For this review, take the finished solid that the model builds, in its own axes (mm). Face numbers are marked on the shaded views. Coordinates: 2 decimals unless noted, no trailing zeros. Loops run counter-clockwise (first coordinate to the right, second up) from the corner with the lowest first, then second, coordinate; pieces in that order, holes last. Notation, with made-up numbers: (-2, 40.25) - (51, 40.25) arc R23 ccw to (51, 49.25) - close; hole circle Ø3 at (30.5, 49.25). An arc over 180 degrees is marked (long way). Answer as a JSON object with one key per item and string values. Group by question number.
Item 1: We need section A-A (x = 0.4). Give the boundary of the cut face in (y, z).
Item 2: Clearance check with flat-ended pins moving along their axes: pin 1 (1.9 mm diameter, centred on y = 8, z = 90, fed in from -X); pin 2 (2 mm diameter, centred on x = 2.5, y = 0.5, fed in from -Z). State where each tip first meets the part, or that it passes through.
Item 3: We need section C-C (z = 108). Give the boundary of the cut face in (x, y), then the cut area to 3 significant figures.
Item 4: To check wall thickness, follow line 1 (Z direction, x = 3.1, y = 9); line 2 (Z direction, x = 2.05, y = 8); line 3 (Y direction, x = 1.2, z = 108). State the ranges of each line that lie inside material, in increasing order.
Item 5: Mouldability with a two-part tool opening along Y and no side actions: class the marked faces 1, 2 and 3 as released by +Y, released by -Y, zero draft, split by the parting line, or undercut.
Item 6: We need section B-B (y = 8). Give the boundary of the cut face in (x, z).
Item 7: We need section D-D (y = 2.5). Give the boundary of the cut face in (x, z).
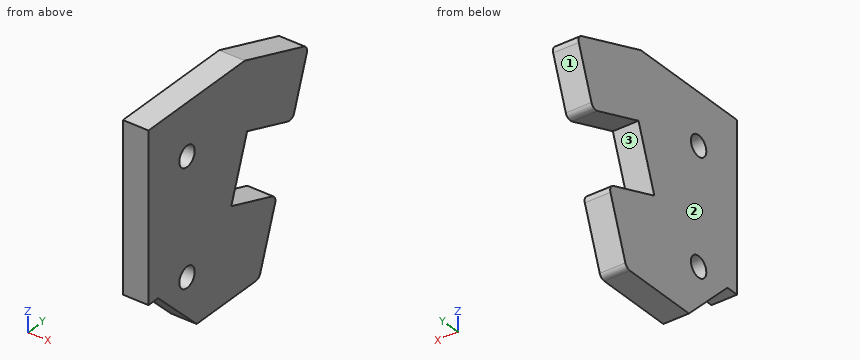
Autodesk Fusion 360 part; units mm, degrees
sketch "スケッチ1" plane through (0, 0, 0) normal (1, 0, 0) x (0, 0, -1)
  line L0 (-116, 0) -> (-116, 20)
  line L1 (-116, 20) -> (-111.3943, 33.2207)
  line L2 (-111.3943, 33.2207) -> (-101.951, 29.931)
  line L3 (-101.951, 29.931) -> (-105.2407, 20.4876)
  line L4 (-105.2407, 20.4876) -> (-95.7973, 17.1978)
  line L5 (-14, 252) -> (0, 252)
  line L6 (-95.7973, 17.1978) -> (-79.3485, 64.4147)
  line L7 (-79.3485, 64.4147) -> (-65.1834, 59.4801)
  line L8 (-65.1834, 59.4801) -> (-63.8675, 63.2574)
  line L9 (-63.8675, 63.2574) -> (-78.0326, 68.1921)
  line L10 (-78.0326, 68.1921) -> (-38.5555, 181.5127)
  line L11 (-38.5555, 181.5127) -> (-24.3904, 176.578)
  line L12 (-24.3904, 176.578) -> (-23.0745, 180.3554)
  line L13 (-23.0745, 180.3554) -> (-37.2396, 185.29)
  line L14 (-37.2396, 185.29) -> (-14, 252)
  line L15 (-116, 0) -> (-70, 0)
  line L16 (-70, 0) -> (-70, -4)
  line L17 (-70, -4) -> (-50, -4)
  line L18 (-50, -4) -> (-50, 0)
  line L19 (-50, 0) -> (0, 0)
  line L20 (0, 252) -> (0, 165)
  line L21 (0, 165) -> (4, 165)
  line L22 (4, 165) -> (4, 145)
  line L23 (4, 145) -> (0, 145)
  line L24 (0, 145) -> (0, 0)
  line L25 (4, 155) -> (-13.5, 155)
  line L26 (-60, -4) -> (-60, 13.5)
  line L27 (-64.1481, 77.6509) -> (-33.5533, 165.4743)
  line L28 (-10, 10) -> (-30, 10)
  line L29 (-30, 10) -> (-30, 30)
  line L30 (-30, 30) -> (-10, 30)
  line L31 (-10, 30) -> (-10, 10)
  line L32 (-108, 8) -> (-90, 8)
  line L33 (-102.8799, 19.6651) -> (-98.1582, 18.0203)
  line L34 (-98.1582, 18.0203) -> (-99.1451, 15.1873)
  line L35 (-99.1451, 15.1873) -> (-103.8668, 16.8321)
  line L36 (-103.8668, 16.8321) -> (-102.8799, 19.6651)
  line L37 (-92.5076, 26.6412) -> (-82, 22.9807)
  line L38 (-82, 22.9807) -> (-82, 0)
  line L39 (-90, 0) -> (-90, 2)
  line L40 (-90, 2) -> (-82, 10)
  dimension "d1" = 116
  dimension "d2" = 20
  dimension "d3" = 14
  dimension "d4" = 10
  dimension "d5" = 10
  dimension "d6" = 10
  dimension "d9" = 14
  dimension "d11" = 252
  dimension "d12" = 248.642
  dimension "d13" = 4
  dimension "d14" = 4
  dimension "d15" = 120
  dimension "d16" = 50
  dimension "d17" = 15
  dimension "d18" = 20
  dimension "d19" = 4
  dimension "d20" = 50
  dimension "d21" = 4
  dimension "d22" = 20
  dimension "d23" = 145
  dimension "d24" = 17.5
  dimension "d25" = 17.5
  dimension "d31" = 10
  dimension "d32" = 13.5
  dimension "d33" = 13.5
  dimension "d36" = 10
  dimension "d37" = 20
  dimension "d38" = 20
  dimension "d39" = 10
  dimension "d40" = 8
  dimension "d41" = 8
  dimension "d42" = 18
  dimension "d43" = 5
  dimension "d44" = 3
  dimension "d45" = 34
  dimension "d46" = 135
  dimension "d47" = 2
  dimension "d48" = 8
extrude "押し出し1" add sketch "スケッチ1" along normal blind 4 contours L0 L1 L2 L3 L4 L6 L15 L34 L35 L36 L37 L38 L39 L40 | L4 L33 L34 L35 L36
hole "穴1" at (0, 8, 90) at (0, 8, 108) direction (1, 0, 0) diameter 3.2 end through all
fillet "フィレット1" radius 1 4 edges at (2, 29.931, 101.951) (2, 33.2207, 111.3943) (2, 26.6412, 92.5076) (2, 22.9807, 82)
Check sheet entries:
{
 "1": {"outline": "(0, 90) - (2, 90) - (10, 82) - (22.27, 82) arc R1 ccw to (23.21, 82.67) - (26.31, 91.56) arc R1 ccw to (25.7, 92.84) - (17.2, 95.8) - (20.49, 105.24) - (28.99, 102.28) arc R1 ccw to (30.26, 102.9) - (32.89, 110.45) arc R1 ccw to (32.28, 111.72) - (20, 116) - (0, 116) - close; hole circle Ø3.2 at (8, 90); hole circle Ø3.2 at (8, 108)"},
 "2": {"pin 1": "passes through", "pin 2": "stops at z = 90"},
 "3": {"outline": "(0, 0) - (4, 0) - (4, 6.4) - (0, 6.4) - close; (0, 9.6) - (4, 9.6) - (4, 32.04) - (0, 32.04) - close", "area": "115 mm2"},
 "4": {"line 1": "z = 83 to 88.75, 91.25 to 106.75, 109.25 to 116", "line 2": "z = 84 to 88.4, 91.6 to 106.4, 109.6 to 116", "line 3": "y = 0 to 6.4, 9.6 to 32.04"},
 "5": {"face 1": "released by +Y", "face 2": "zero draft", "face 3": "undercut"},
 "6": {"outline": "(0, 84) - (4, 84) - (4, 88.4) - (0, 88.4) - close; (0, 91.6) - (4, 91.6) - (4, 106.4) - (0, 106.4) - close; (0, 109.6) - (4, 109.6) - (4, 116) - (0, 116) - close"},
 "7": {"outline": "(0, 89.5) - (4, 89.5) - (4, 116) - (0, 116) - close"}
}
